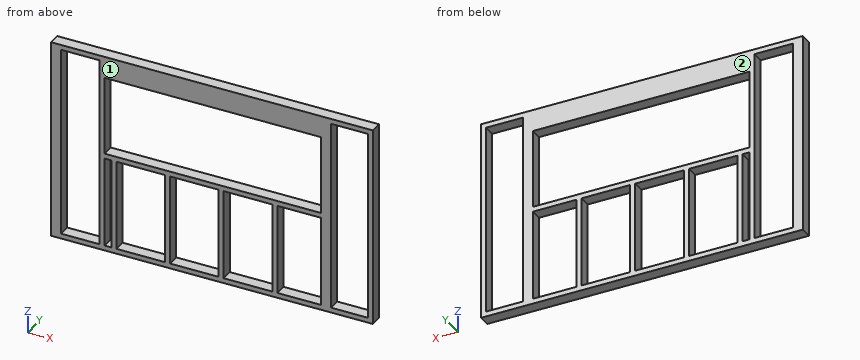
```python
from build123d import *

# Parameters (mm, degrees)
F0_W     = 2438.4
F0_H     = 88.9
F1_DEPTH = 38.1
F2_W     = 38.1
F2_H     = 88.9
F3_DEPTH = 1447.8
F4_W     = 2438.4
F4_H     = 38.1
F5_DEPTH = 88.9
F7_DEPTH = 88.9
F8_W     = 1638.3
F8_H     = 596.9
F9_DEPTH = 215.9


with BuildPart() as f1:
    # F0 (on Top) → F1 (new body)
    with BuildSketch(Plane.XY):
        Rectangle(F0_W, F0_H)
    extrude(amount=F1_DEPTH)

    # F2 (on face) → F3 (join)
    with BuildSketch(Plane.XY.offset(38.1)):
        with Locations((1200.15, 0)):
            Rectangle(F2_W, F2_H)
        with Locations((882.65, 0)):
            Rectangle(F2_W, F2_H)
        with Locations((476.25, 0)):
            Rectangle(F2_W, F2_H)
        with Locations((69.85, 0)):
            Rectangle(F2_W, F2_H)
        with Locations((-336.55, 0)):
            Rectangle(F2_W, F2_H)
        with Locations((-742.95, 0)):
            Rectangle(F2_W, F2_H)
        with Locations((-1200.15, 0)):
            Rectangle(F2_W, F2_H)
        with Locations((-1162.05, 0)):
            Rectangle(F2_W, F2_H)
    extrude(amount=F3_DEPTH)

    # F4 (on face) → F5 (join)
    with BuildSketch(Plane(origin=(0, 44.45, 0), x_dir=(-1, 0, 0), z_dir=(0, 1, 0))):
        with Locations((0, 1504.95)):
            Rectangle(F4_W, F4_H)
    extrude(amount=-F5_DEPTH)

    # F6 (on face) → F7 (join)
    with BuildSketch(Plane.XZ.offset(44.45)):
        Polygon((825.5, 762), (812.8, 762), (-812.8, 762), (-812.8, 723.9), (825.5, 723.9), align=None)
        Polygon((-812.8, 723.9), (-812.8, 762), (-812.8, 1358.9), (-812.8, 1485.9), (-850.9, 1485.9), (-850.9, 38.1), (-812.8, 38.1), align=None)
        Polygon((-812.8, 1358.9), (812.8, 1358.9), (825.5, 1358.9), (825.5, 1485.9), (-812.8, 1485.9), align=None)
        Polygon((825.5, 1358.9), (825.5, 762), (825.5, 723.9), (825.5, 38.1), (863.6, 38.1), (863.6, 1485.9), (825.5, 1485.9), align=None)
    extrude(amount=-F7_DEPTH)

    # F8 (on face) → F9 (cut)
    with BuildSketch(Plane.XZ.offset(44.45)):
        with Locations((6.35, 1060.45)):
            Rectangle(F8_W, F8_H)
    extrude(amount=-F9_DEPTH, mode=Mode.SUBTRACT)


solid = f1.part
```
Can you work these out from the model? Positions are in its coordinate system, mm. Face numbers are marked on the shaded views. Give positions to 0.01 mm unless a question says otherwise; leave off trailing zeros. Write each loop counter-clockwise with the first axis right and the second up, starting at its lowest first coordinate (ties: lowest second). Pieces come first, ordered by that corner, then holes. Notation, with made-up numbers: (57, 83) -> (103, 83) arc R20 ccw to (103, 100) -> close; hole circle Ø6 at (1.5, 82.5). An arc over 180 degrees is marked (long way). One line per item, written item: value.
Q1. Please list where these lines run through material, in increasing order: line 1 (Z direction, x = -667, y = 38.5); line 2 (X direction, y = 31, z = 1266); line 3 (X direction, y = 10, z = 1360.5). Write a range as [from, to].
Results found:
line 1: z = [0, 38.1], [723.9, 762], [1358.9, 1524]
line 2: x = [-1219.2, -1143], [-850.9, -812.8], [825.5, 901.7], [1181.1, 1219.2]
line 3: x = [-1219.2, -1143], [-850.9, 901.7], [1181.1, 1219.2]
Q2. Imagine slicing it at D-D on z = 1277.5. Please give me the cut outline in (x, y).
Results found:
outline: (-1219.2, -44.45) -> (-1143, -44.45) -> (-1143, 44.45) -> (-1219.2, 44.45) -> close; (-850.9, -44.45) -> (-812.8, -44.45) -> (-812.8, 44.45) -> (-850.9, 44.45) -> close; (825.5, -44.45) -> (901.7, -44.45) -> (901.7, 44.45) -> (825.5, 44.45) -> close; (1181.1, -44.45) -> (1219.2, -44.45) -> (1219.2, 44.45) -> (1181.1, 44.45) -> close
Q3. Imagine slicing it at A-A on x = 1029. Please give me the cut outline in (y, z).
Results found:
outline: (-44.45, 0) -> (44.45, 0) -> (44.45, 38.1) -> (-44.45, 38.1) -> close; (-44.45, 1485.9) -> (44.45, 1485.9) -> (44.45, 1524) -> (-44.45, 1524) -> close
Q4. For P1, Ø4, axis at x = 681.5, y = -16, coming from the -Z side, with a flat end and sliding along its axis, tell me the tip position at first contact or that it passes through.
Results found:
P1: stops at z = 0
Q5. We'd pull the mould along Y, two halves only. Please class the marked faces 1 and 2: +Y half, -Y half, draft (parallel to the pull), parting line (faces both ways), or undercut.
Results found:
face 1: -Y half
face 2: +Y half
Q6. Imagine slicing it at B-B on z = 474. Give the number of separate pieces and of enclosed holes in the cut face, and give its area (3 significant figures).
Results found:
separate pieces: 8
enclosed holes: 0
area: 33,900 mm^2
Q7. Imagine slicing it at C-C on x = 174. Please give me the cut outline in (y, z), and give its area (3 significant figures).
Results found:
outline: (-44.45, 0) -> (44.45, 0) -> (44.45, 38.1) -> (-44.45, 38.1) -> close; (-44.45, 723.9) -> (44.45, 723.9) -> (44.45, 762) -> (-44.45, 762) -> close; (-44.45, 1358.9) -> (44.45, 1358.9) -> (44.45, 1524) -> (-44.45, 1524) -> close
area: 21,500 mm^2
